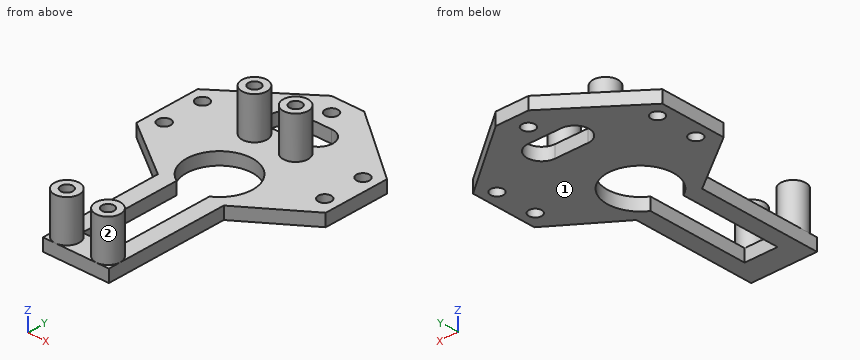
from build123d import *

# Parameters (mm, degrees)
SKETCH_R     = 1.55
PAD_DEPTH    = 3
SKETCH001_R  = 3
PAD001_DEPTH = 10
SKETCH002_R  = 1.45
POCKET_DEPTH = 7


with BuildPart() as part:
    # Sketch → Pad (new body)
    with BuildSketch(Plane.XY):
        Polygon((8, -30), (-8, -30), (-8, 0), (-23, 10.503113), (-23, 26.503113), (-4, 41), (4, 41), (23, 26.503113), (23, 10.503113), (8, 0), align=None)
        with Locations((0, 36.75)):
            Circle(SKETCH_R, mode=Mode.SUBTRACT)
        with Locations((19.5, 24)):
            Circle(SKETCH_R, mode=Mode.SUBTRACT)
        with Locations((19.5, 14)):
            Circle(SKETCH_R, mode=Mode.SUBTRACT)
        with Locations((-19.5, 24)):
            Circle(SKETCH_R, mode=Mode.SUBTRACT)
        with Locations((-19.5, 14)):
            Circle(SKETCH_R, mode=Mode.SUBTRACT)
        with BuildLine():
            ThreePointArc((-4, 32.5), (-7.5, 29), (-4, 25.5))
            Line((-4, 25.5), (4, 25.5))
            ThreePointArc((4, 25.5), (7.5, 29), (4, 32.5))
            Line((-4, 32.5), (4, 32.5))
        make_face(mode=Mode.SUBTRACT)
        with BuildLine():
            ThreePointArc((4, 0.571797), (0, 15.5), (-4, 0.571797))
            Line((-4, -24), (-4, 0.571797))
            Line((4, -24), (-4, -24))
            Line((4, 0.571797), (4, -24))
        make_face(mode=Mode.SUBTRACT)
    extrude(amount=PAD_DEPTH)

    # Sketch001 (on Face25 of Pad) → Pad001 (join)
    with BuildSketch(Plane.XY.offset(3)):
        with Locations((-5, 22)):
            Circle(SKETCH001_R)
        with Locations((5, 22)):
            Circle(SKETCH001_R)
        with Locations((5, -27)):
            Circle(SKETCH001_R)
        with Locations((-5, -27)):
            Circle(SKETCH001_R)
    extrude(amount=PAD001_DEPTH)

    # Sketch002 (on Face35 of Pad001) → Pocket (cut)
    with BuildSketch(Plane.XY.offset(13)):
        with Locations((-5, 22)):
            Circle(SKETCH002_R)
        with Locations((5, 22)):
            Circle(SKETCH002_R)
        with Locations((5, -27)):
            Circle(SKETCH002_R)
        with Locations((-5, -27)):
            Circle(SKETCH002_R)
    extrude(amount=-POCKET_DEPTH, mode=Mode.SUBTRACT)


solid = part.part
Design review of the part built by this model. Coordinates are the model's own, in mm. Face numbers are marked on the shaded views. Round coordinates to 2 decimals unless told otherwise and drop trailing zeros. Loops run counter-clockwise (first coordinate to the right, second up) from the corner with the lowest first, then second, coordinate; pieces in that order, holes last. Notation, with made-up numbers: (55.25, -13) - (73.25, -13) arc R20 ccw to (73.25, 26) - close; hole circle Ø7 at (-23, -8). An arc over 180 degrees is marked (long way). One line per question, with ' | ' between items.
1. We need section A-A, the plane x = 0. State the section outline as (y, z) points.
Results are:
outline: (-30, 0) - (-24, 0) - (-24, 3) - (-30, 3) - close; (15.5, 0) - (25.5, 0) - (25.5, 3) - (15.5, 3) - close; (32.5, 0) - (35.2, 0) - (35.2, 3) - (32.5, 3) - close; (38.3, 0) - (41, 0) - (41, 3) - (38.3, 3) - close
2. For L1, parallel to Y at x = -5, z = 10.75; L2, parallel to Y at x = -4, z = 12.25; L3, parallel to X at y = 9.5, z = 2.5, list the stretches that pass through material, from the lowest coordinate up. Write a range as [from, to].
Results are:
L1: y = [-30, -28.45], [-25.55, -24], [19, 20.55], [23.45, 25] | L2: y = [-29.83, -28.05], [-25.95, -24.17], [19.17, 20.95], [23.05, 24.83] | L3: x = [-21.57, -7.75], [7.75, 21.57]
3. Draft analysis for pull direction Y (two halves, no side actions). For the marked faces 1 and 2, state which applies: released by +Y, released by -Y, zero draft, split by the parting line, or undercut.
Results are:
face 1: zero draft | face 2: undercut
4. Clearance check with flat-ended pins moving along their axes: P1, Ø2.5, axis at x = 5, y = 22, coming from the +Z side; P2, Ø0.9, axis at y = -11, z = 1.5, coming from the -X side; P3, Ø3, axis at x = -19.5, y = 24, coming from the -Z side; P4, Ø1.5, axis at y = -9, z = 2, coming from the +X side. State where each tip first meets the part, or that it passes through.
Results are:
P1: stops at z = 6 | P2: stops at x = -8 | P3: passes through | P4: stops at x = 8
5. We need section B-B, the plane z = 11. State the section outline as (x, y) points, and give its area (3 significant figures).
Results are:
outline: circle Ø6 at (-5, -27); circle Ø6 at (-5, 22); circle Ø6 at (5, -27); circle Ø6 at (5, 22); hole circle Ø2.9 at (-5, -27); hole circle Ø2.9 at (-5, 22); hole circle Ø2.9 at (5, -27); hole circle Ø2.9 at (5, 22) | area: 86.7 mm²
6. We need section D-D, the plane z = 1.5. State the section outline as (x, y) points, and give its area (3 significant figures).
Results are:
outline: (-23, 10.5) - (-8, 0) - (-8, -30) - (8, -30) - (8, 0) - (23, 10.5) - (23, 26.5) - (4, 41) - (-4, 41) - (-23, 26.5) - close; hole circle Ø3.1 at (-19.5, 14); hole circle Ø3.1 at (-19.5, 24); hole (-4, -24) - (4, -24) - (4, 0.57) arc R8 ccw (long way) to (-4, 0.57) - close; hole (-4, 25.5) - (4, 25.5) arc R3.5 ccw to (4, 32.5) - (-4, 32.5) arc R3.5 ccw to start; hole circle Ø3.1 at (0, 36.75); hole circle Ø3.1 at (19.5, 14); hole circle Ø3.1 at (19.5, 24) | area: 1,410 mm²
7. We need section C-C, the plane y = 14. State the section outline as (x, z) points, and give its area (3 significant figures).
Results are:
outline: (-23, 0) - (-21.05, 0) - (-21.05, 3) - (-23, 3) - close; (-17.95, 0) - (-4.66, 0) - (-4.66, 3) - (-17.95, 3) - close; (4.66, 0) - (17.95, 0) - (17.95, 3) - (4.66, 3) - close; (21.05, 0) - (23, 0) - (23, 3) - (21.05, 3) - close | area: 91.4 mm²
